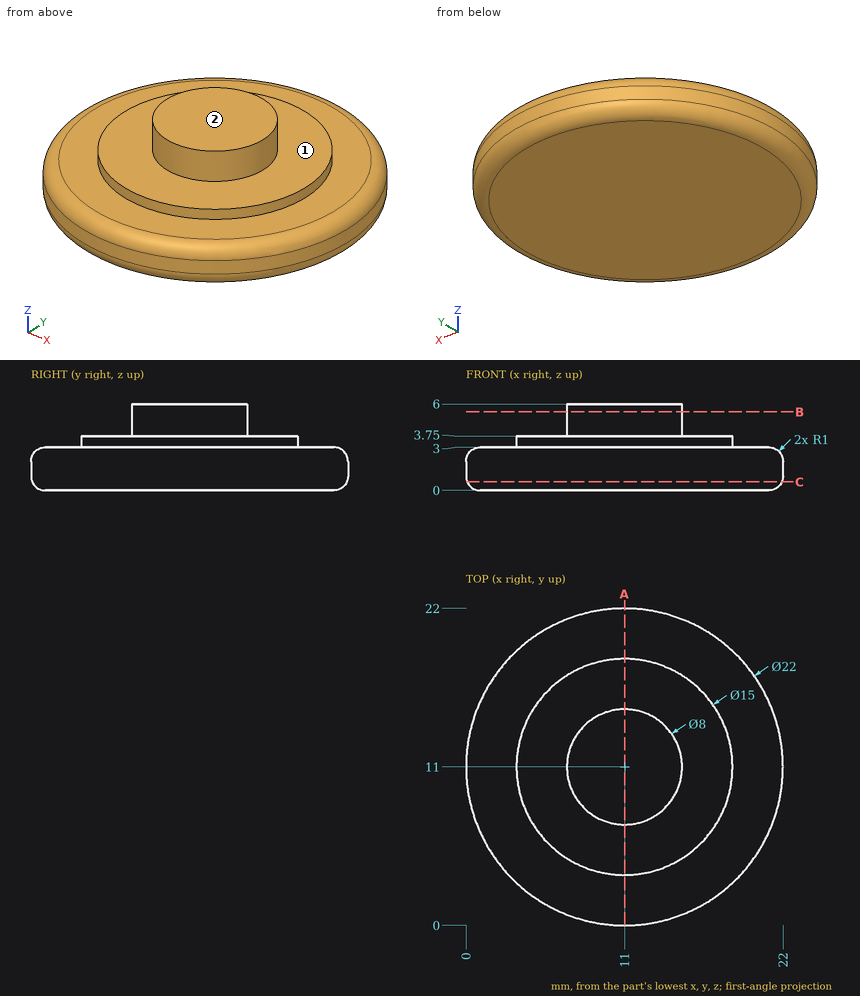
Geometry check sheet. Reference: drawing and pictorial views, mm from the part's lowest x, y, z. A direction names the side the tool comes from. Round coordinates to 2 decimals unless told otherwise and drop trailing zeros. Write each loop counter-clockwise with the first axis right and the second up, starting at its lowest first coordinate (ties: lowest second). Pieces come first, ordered by that corner, then holes.
(1) Section check C-C (z = 0.6). Enter the section's corners in (x, y), plus the area to 3 significant figures.
Returned:
outline: circle Ø21.83 at (11, 11)
area: 374 mm2
(2) Section check A-A (x = 11). Enter the section's corners in (y, z), plus the area to 3 significant figures.
Returned:
outline: (0, 1) arc R1 ccw to (1, 0) - (21, 0) arc R1 ccw to (22, 1) - (22, 2) arc R1 ccw to (21, 3) - (18.5, 3) - (18.5, 3.75) - (15, 3.75) - (15, 6) - (7, 6) - (7, 3.75) - (3.5, 3.75) - (3.5, 3) - (1, 3) arc R1 ccw to (0, 2) - close
area: 94.4 mm2
(3) Access from +Z, -Z, +X, -X, +Y, -Y to the whole of each face (thin tool, end or side, straight path). Record for the marked faces 1 and 2.
Returned:
face 1: +Z
face 2: +Z, +X, -X, +Y, -Y
(4) Section check B-B (z = 5.45). Enter the section's corners in (x, y), plus the area to 3 significant figures.
Returned:
outline: circle Ø8 at (11, 11)
area: 50.3 mm2
(5) Material ranges on line 1 (Z direction, x = 6.75, y = 20); line 2 (Z direction, x = 16.25, y = 12.5); line 3 (Y direction, x = 12.25, z = 1.25), recorded low to high.
Returned:
line 1: z = 0 to 3
line 2: z = 0 to 3.75
line 3: y = 0.07 to 21.93
(6) Depth check by flat-ended pin: pin 1 Ø3 at (x, z) = (6.5, 2.5) entering from -Y; pin 2 Ø2 at (y, z) = (15, 3) entering from +X. Enter the tip coordinate at first touch or a pass-through.
Returned:
pin 1: stops at y = 0.44
pin 2: stops at x = 21.45
